```python
from build123d import *

# Parameters (mm, degrees)
F0_W     = 55.56523
F0_H     = 44.569992
F1_DEPTH = 25.4
F2_R     = 5.218262
F3_DEPTH = 110.220805


with BuildPart() as f1:
    # F0 (on Front) → F1 (new body)
    with BuildSketch(Plane.XZ):
        Rectangle(F0_W, F0_H)
    extrude(amount=F1_DEPTH)

    # F2 (on Top) → F3 (join)
    with BuildSketch(Plane.XY):
        with Locations((0, -10.700724)):
            Circle(F2_R)
    extrude(amount=-F3_DEPTH)


solid = f1.part
```
The model under review builds one solid part; all positions refer to its coordinate system, in mm. A direction names the side the tool comes from. Round coordinates to 2 decimals unless told otherwise and drop trailing zeros. Write each loop counter-clockwise with the first axis right and the second up, starting at its lowest first coordinate (ties: lowest second). Pieces come first, ordered by that corner, then holes.
(1) We need section C-C on y = -21. Give the boundary of the cut face in (x, z) (3 decimals), and give its area (3 significant figures).
(2) We need section D-D on z = -36.5. Give the boundary of the cut face in (x, y).
(3) We need section B-B on y = -6.75. Give the boundary of the cut face in (x, z) (3 decimals), and give its area (3 significant figures).
(4) Machinability: for faces 1 (the cylindrical face through (-1.1, -15.8, -65.6)), 2 (the flat face through (27.783, -13, 0)), which of the approach directions +Z, -Z, +X, -X, +Y, -Y give a long, thin tool a straight path to every point of the face, cutting with its end or side? Answer none if there is none.
(5) We need section A-A on x = 0. Give the boundary of the cut face in (y, z) (3 decimals), and give its area (3 significant figures).
(6) Insertion check: pin 1 (12.5 mm diameter, centred on x = 12.5, y = -18, fed in from -Z) (3 decimals). The pin has a flat end and moves straight along its axis. Give the tip position at first contact, or say it passes through.
(7) Wall thickness on L1, parallel to Z at x = 10, y = -22.75 (3 decimals); L2, parallel to X at y = -9.75, z = -97; L3, parallel to X at y = -10, z = -100.5: over which ranges is each line inside the solid? List them lowest first.
Findings below:
1. outline: (-27.783, -22.285) - (27.783, -22.285) - (27.783, 22.285) - (-27.783, 22.285) - close
1. area: 2,480 mm2
2. outline: circle Ø10.44 at (0, -10.7)
3. outline: (-27.783, -22.285) - (-3.409, -22.285) - (-3.409, -110.221) - (3.409, -110.221) - (3.409, -22.285) - (27.783, -22.285) - (27.783, 22.285) - (-27.783, 22.285) - close
3. area: 3,080 mm2
4. face 1: -Z
4. face 2: +Z, -Z, +X, +Y, -Y
5. outline: (-25.4, -22.285) - (-15.919, -22.285) - (-15.919, -110.221) - (-5.482, -110.221) - (-5.482, -22.285) - (0, -22.285) - (0, 22.285) - (-25.4, 22.285) - close
5. area: 2,050 mm2
6. pin 1: stops at z = -22.285
7. L1: z = -22.285 to 22.285
7. L2: x = -5.13 to 5.13
7. L3: x = -5.17 to 5.17
